For this review, use the dimensioned drawing (mm, ordinates from the lowest corner) and the shaded views. Round coordinates to 2 decimals unless told otherwise and drop trailing zeros. Order: outer loops, then holes, each group sorted by start corner. A loop starts at its lowest first (then second) coordinate and runs counter-clockwise, first axis right, second up. Notation, with made-up numbers: (-0.5, 13.25) - (9.5, 13.25) arc R27 ccw to (9.5, 35.25) - close; hole circle Ø5 at (13, 33). An arc over 180 degrees is marked (long way). Write item = value, one per line.
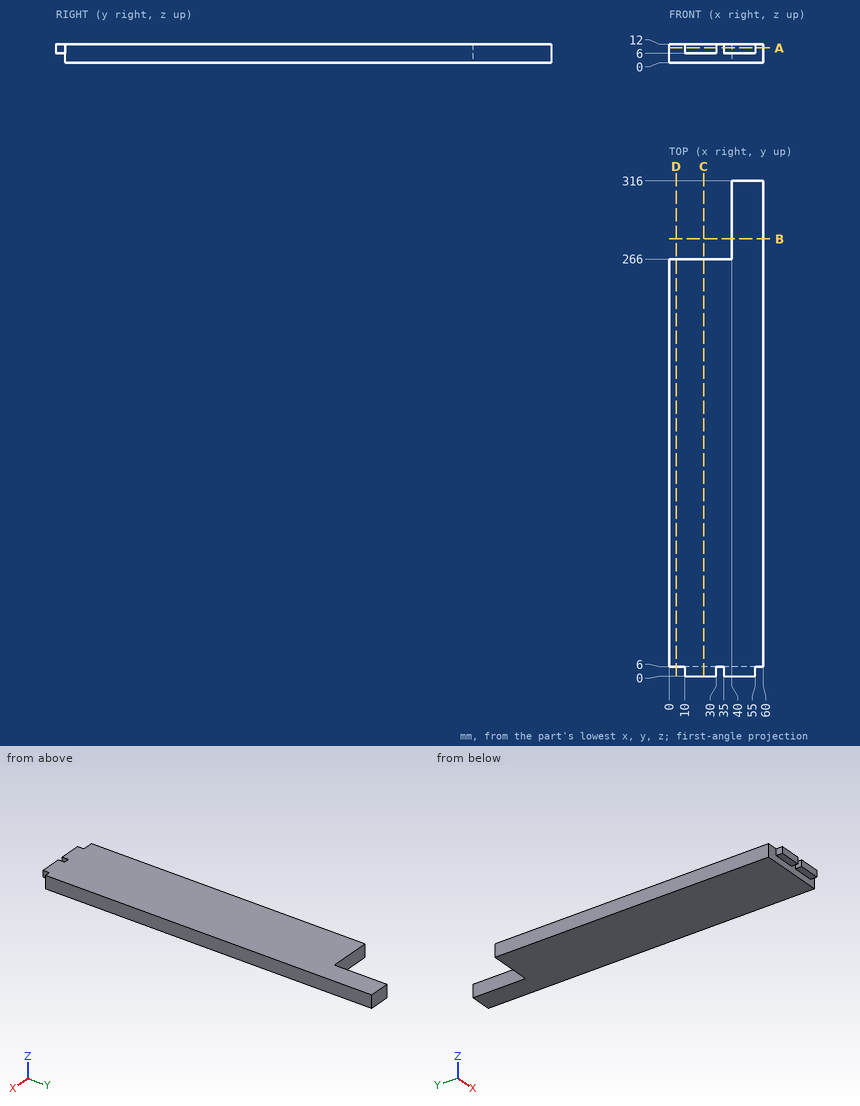
Item 1: Take a section at C-C, the plane x = 22. State the section outline as (y, z) points, and give its area (3 significant figures).
Data:
outline = (0, 6) - (6, 6) - (6, 0) - (266, 0) - (266, 12) - (0, 12) - close
area = 3,160 mm2
Item 2: Insertion check: P1, Ø3, axis at y = 2, z = 10, coming from the -X side; P2, Ø1.8, axis at y = 4, z = 7.5, coming from the +X side; P3, Ø6, axis at y = 284, z = 4, coming from the -X side. Each pin has a flat end and moves straight along its axis. Give the tip position at first contact, or say it passes through.
Data:
P1 = 10
P2 = 55
P3 = 40
Item 3: Take a section at B-B, the plane y = 279. State the section outline as (x, z) points, and give its area (3 significant figures).
Data:
outline = (40, 0) - (60, 0) - (60, 12) - (40, 12) - close
area = 240 mm2
Item 4: Take a section at D-D, the plane x = 4.5. State the section outline as (y, z) points.
Data:
outline = (6, 0) - (266, 0) - (266, 12) - (6, 12) - close
Item 5: Take a section at A-A, the plane z = 9.5. State the section outline as (x, y) points, and give its area (3 significant figures).
Data:
outline = (0, 6) - (10, 6) - (10, 0) - (30, 0) - (30, 6) - (35, 6) - (35, 0) - (55, 0) - (55, 6) - (60, 6) - (60, 316) - (40, 316) - (40, 266) - (0, 266) - close
area = 16,800 mm2
Item 6: For line 1 along Y through (x, z) = (21.5, 1.5); line 2 along Y through (x, z) = (51, 3), list the stretches that pass through material, from the lowest coordinate up. Write a range as [from, to].
Data:
line_1 = [6, 266]
line_2 = [6, 316]
